Can you work these out from the model? Positions are in its coordinate system, mm. Face numbers are marked on the shaded views. Coordinates: 2 decimals unless noted, no trailing zeros. Loops run counter-clockwise (first coordinate to the right, second up) from the corner with the lowest first, then second, coordinate; pieces in that order, holes last. Notation, with made-up numbers: (2, 80) -> (18, 80) arc R19 cw to (18, 100) -> close; hole circle Ø4 at (-22, 48.25). An arc over 180 degrees is marked (long way). Put each result on its own line as item: value. Start each with the question number.
Item 1: If we section it at C-C on z = 5.25: State how many separate pieces and enclosed holes the cut face has, plus the area to 3 significant figures.
Item 2: If we section it at A-A on x = 1010: Please give me the cut outline in (y, z) (3 decimals), plus the area to 3 significant figures.
Item 3: We'd pull the mould along Z, two halves only. Please class the marked faces 1 and 2: pulls with the +Z half, pulls with the -Z half, needs draft (parallel to the pull), parting line crosses it, or undercut.
Item 4: If we section it at B-B on y = 115: Please give me the cut outline in (x, z).
Item 5: Please list where these lines run through material, in increasing order: L1, parallel to Y at x = 953, z = 5; L2, parallel to Y at x = 1003.5, z = 4.25; L3, parallel to X at y = 145, z = 6. Write a range as from..to.
Item 6: Will these pins go through, and if not, where does the flat tip stop? P1, Ø5.5, axis at x = 880.54, y = 617.91, coming from the +Z side; P2, Ø5.5, axis at y = -243.5, z = 13, coming from the +X side; P3, Ø4, axis at x = 680, z = 13, coming from the +Y side; P4, Ø4, axis at y = 413, z = 6.5, coming from the +X side.
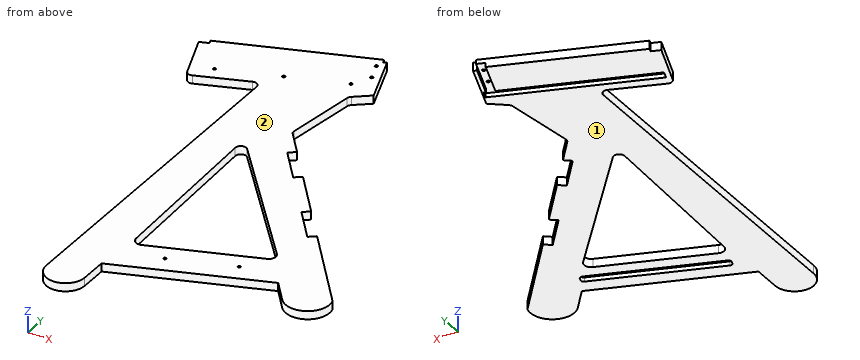
```python
from build123d import *

# Parameters (mm, degrees)
F1_DEPTH = 19.05
F3_DEPTH = 9.525
F5_DEPTH = 9.525
F6_W     = 94.742
F6_H     = 19.05
F6_H_2   = 22.0252738774
F7_DEPTH = 19.558
F8_R     = 3.302
F9_DEPTH = 19.051


# Not quite as in the source:
# - a feature names something its author has since deleted; it is built from what else it names


with BuildPart() as f1:
    # F0 (on Top) → F1 (new body)
    with BuildSketch(Plane.XY):
        with BuildLine():
            Line((727.2677384075, 427.9083177516), (727.2677384075, -283.5772421425))
            ThreePointArc((727.2677384075, -283.5772421425), (771.8616098047, -328.1711135397), (816.4554812019, -283.5772421425))
            Line((816.4554812019, -283.5772421425), (816.4554812019, -220.0584400703))
            Line((816.4554812019, -220.0584400703), (1153.129473529, -100.186362138))
            Line((1153.129473529, -100.186362138), (1192.5444383312, -149.4502630935))
            ThreePointArc((1192.5444383312, -149.4502630935), (1256.128693756, -162.5951765711), (1280.8355912672, -102.5508970465))
            Line((1280.8355912672, -102.5508970465), (881.2480453078, 396.8848219998))
            ThreePointArc((881.2480453078, 396.8848219998), (878.9075846932, 401.4943033077), (878.5980767553, 406.6546597539))
            Line((878.5980767553, 406.6546597539), (902.2401524871, 568.497452094))
            ThreePointArc((902.2401524871, 568.497452094), (903.8120375637, 573.0182606597), (906.9455405898, 576.6362285378))
            Line((906.9455405898, 576.6362285378), (941.9003890149, 604.1852707886))
            Line((941.9003890149, 604.1852707886), (899.3018677789, 723.8279303566))
            Line((899.3018677789, 723.8279303566), (891.7270738587, 721.1309406639))
            Line((891.7270738587, 721.1309406639), (888.532184766, 730.1041401315))
            Line((888.532184766, 730.1041401315), (557.8398737201, 612.361827435))
            Line((557.8398737201, 612.361827435), (561.0347628128, 603.3886279674))
            Line((561.0347628128, 603.3886279674), (540.3738890749, 596.0323666485))
            Line((540.3738890749, 596.0323666485), (579.864860977, 488.7712220609))
            ThreePointArc((579.864860977, 488.7712220609), (586.4582383014, 481.6291726364), (596.1706516981, 481.2412028737))
            Line((596.1706516981, 481.2412028737), (710.1798391165, 523.2166417359))
            ThreePointArc((710.1798391165, 523.2166417359), (721.8328511307, 521.7154565085), (727.2677384075, 511.2987273493))
            Line((727.2677384075, 511.2987273493), (727.2677384075, 427.9083177516))
        make_face()
        with BuildLine():
            ThreePointArc((847.13107515, -119.4008734987), (832.2962861388, -117.4908698033), (825.0919590872, -104.3829809246))
            Line((825.0919590872, -104.3829809246), (812.2279623998, 291.9047427935))
            ThreePointArc((812.2279623998, 291.9047427935), (820.3847868922, 304.1789193457), (834.6503380579, 300.4798321914))
            Line((834.6503380579, 300.4798321914), (1093.5127410116, -8.0431735903))
            ThreePointArc((1093.5127410116, -8.0431735903), (1096.7972352344, -22.9844248457), (1086.4027687189, -34.2086823816))
            Line((1086.4027687189, -34.2086823816), (847.13107515, -119.4008734987))
        make_face(mode=Mode.SUBTRACT)
    extrude(amount=F1_DEPTH)

    # F2 (on face) → F3 (cut)
    with BuildSketch(Plane.XY):
        with BuildLine():
            ThreePointArc((844.1222933391, -166.9052020902), (847.3560158569, -170.6500208272), (852.2954479263, -170.9374917442))
            Line((852.2954479263, -170.9374917442), (1129.8610507564, -72.1108335167))
            ThreePointArc((1129.8610507564, -72.1108335167), (1133.425786756, -68.9382065458), (1133.77435322, -64.1788572139))
            Line((1133.77435322, -64.1788572139), (1131.667577719, -57.6492424267))
            ThreePointArc((1131.667577719, -57.6492424267), (1128.4338552012, -53.9044236898), (1123.4944231318, -53.6169527728))
            Line((1123.4944231318, -53.6169527728), (845.9288203018, -152.4436110002))
            ThreePointArc((845.9288203018, -152.4436110002), (842.3640843021, -155.6162379711), (842.0155178382, -160.3755873031))
            Line((842.0155178382, -160.3755873031), (844.1222933391, -166.9052020902))
        make_face()
    extrude(amount=F3_DEPTH, mode=Mode.SUBTRACT)

    # F4 (on face) → F5 (cut)
    with BuildSketch(Plane.XY):
        Polygon((579.9443241227, 521.366756094), (586.5044770697, 502.9417796404), (930.5357275267, 625.4329875525), (924.0377818739, 643.6832473584), (919.8348729601, 642.1868153078), (891.7270738587, 721.1309406639), (888.532184766, 730.1041401315), (870.0541627522, 723.6949228268), (901.3482962404, 635.8015951388), align=None)
    extrude(amount=F5_DEPTH, mode=Mode.SUBTRACT)

    # F6 (on face) → F7 (cut)
    with BuildSketch(Plane(origin=(730.9119602838, 584.7866009261, 0), x_dir=(-0.6247321984, 0.7808390873, 0), z_dir=(0.7808390873, 0.6247321984, 0))):
        with Locations((-357.8801403508, 9.525)):
            Rectangle(F6_W, F6_H)
        with Locations((-584.9891603508, 10.3152221296)):
            Rectangle(F6_W, F6_H_2)
    extrude(amount=-F7_DEPTH, mode=Mode.SUBTRACT)

    # F8 (on face) → F9 (cut, through all)
    with BuildSketch(Plane.XY):
        with Locations((902.6622274527, 660.6120369276)):
            Circle(F8_R)
        with Locations((887.9183335175, 702.107780571)):
            Circle(F8_R)
        with Locations((880.5389518172, 617.9122097817)):
            Circle(F8_R)
        with BuildLine():
            ThreePointArc((623.7483495144, 526.4827509324), (617.3838130375, 524.8132146381), (623.9396392041, 525.3751926427))
            ThreePointArc((623.9396392041, 525.3751926427), (623.8914653707, 525.9371706472), (623.7483495144, 526.4827509324))
        make_face()
        with BuildLine():
            ThreePointArc((756.0284718398, 572.4049919407), (752.1644938352, 575.6588181073), (749.6157615295, 571.2974336509))
            ThreePointArc((749.6157615295, 571.2974336509), (753.2884498444, 569.1511657741), (756.0284718398, 572.4049919407))
        make_face()
        with Locations((1055.4790926394, -88.2571151612)):
            Circle(F8_R)
        with Locations((913.5925848765, -138.7755124943)):
            Circle(F8_R)
    extrude(amount=F9_DEPTH, mode=Mode.SUBTRACT)


solid = f1.part
```
Solutions:
1. separate pieces: 1
1. enclosed holes: 2
1. area: 216,000 mm^2
2. outline: (-151.147, 0) -> (-114.787, 0) -> (-114.787, 9.525) -> (-94.026, 9.525) -> (-94.026, 0) -> (-61.412, 0) -> (-61.412, 19.05) -> (-151.147, 19.05) -> close; (91.491, 0) -> (235.961, 0) -> (235.961, 19.05) -> (91.491, 19.05) -> close
2. area: 4,260 mm^2
3. face 1: pulls with the -Z half
3. face 2: pulls with the +Z half
4. outline: (727.27, 0) -> (817.97, 0) -> (817.97, 19.05) -> (727.27, 19.05) -> close; (990.27, 0) -> (1081.73, 0) -> (1081.73, 19.05) -> (990.27, 19.05) -> close
5. L1: -171.44..-135.08, -114.32..-81.71, 159.43..275.9
5. L2: -153.46..-117.1, -96.34..-63.73, 99.24..244.08
5. L3: 727.27..817, 965.1..1057.73
6. P1: through
6. P2: x = 816.46
6. P3: y = 656.57
6. P4: x = 879.82
